```python
from build123d import *

# Parameters (mm, degrees)
F1_DEPTH = 50
F2_R     = 1.5
F3_DEPTH = 7
F4_R     = 1.5
F5_DEPTH = 7


with BuildPart() as f1:
    # F0 (on Front) → F1 (new body)
    with BuildSketch(Plane.XZ):
        Polygon((-2.165064, 1.25), (0, 0), (0, 2.5), align=None)
        Polygon((2.165064, -1.25), (0, 0), (0, -2.5), align=None)
        Polygon((0, 2.5), (0, 0), (2.165064, 1.25), align=None)
        Polygon((2.165064, 1.25), (0, 0), (2.165064, -1.25), align=None)
        Polygon((0, -2.5), (0, 0), (-2.165064, -1.25), align=None)
        Polygon((-2.165064, -1.25), (0, 0), (-2.165064, 1.25), align=None)
    extrude(amount=F1_DEPTH)

    # F2 (on face) → F3 (join)
    with BuildSketch(Plane.XZ.offset(50)):
        Circle(F2_R)
    extrude(amount=F3_DEPTH)

    # F4 (on face) → F5 (cut)
    with BuildSketch(Plane(origin=(0, 0, 0), x_dir=(-1, 0, 0), z_dir=(0, 1, 0))):
        Circle(F4_R)
    extrude(amount=-F5_DEPTH, mode=Mode.SUBTRACT)


solid = f1.part
```
Build history of the part. All positions in model axes, mm. A direction names the side the tool comes from. Round coordinates to 2 decimals unless told otherwise and drop trailing zeros. Loops run counter-clockwise (first coordinate to the right, second up) from the corner with the lowest first, then second, coordinate; pieces in that order, holes last.
Item 1: Which spindle directions (+Z, -Z, +X, -X, +Y, -Y) get a long thin tool onto all of the face, cutting with end or side? Do faces 1 (the face through (1.5, -3.45, 0.07)), 2 (the face through (-1.5, -53.45, 0.07)), 3 (the face through (1.07, -24.65, -1.88)). Say none if no direction does.
Item 2: Two-plate mould, pull along X, no slides. Class faces 4 (the face through (-1.07, -24.65, 1.88)), 5 (the face through (0, -7, 0)), 6 (the face through (0, -50, -2)): released by +X, released by -X, zero draft, split by the parting line, or undercut.
Item 3: Pin check, flat tip, straight feed: P1, Ø1.8, axis at x = 0, z = 0, coming from the +Y side. Stop position of the tip, or through.
Item 4: Saw through at B-B (y = -6). List the corners of the cut face in (x, z).
Item 5: Saw through at C-C (y = -46.5). List the corners of the cut face in (x, z).
Item 6: Drill centre lines: line 1 along Z through (x, y) = (0, -4.5); line 2 along Y through (x, z) = (0.15, 1.05); line 3 along Y through (x, z) = (0, -2.3). Where is each one in solid material? Low to high.
Item 7: Saw through at D-D (x = -0.9). List the corners of the cut face in (y, z).
Item 8: Saw through at A-A (z = 0). List the corners of the cut face in (x, y).
Worked answers:
1. face 1: +Y
1. face 2: -Y
1. face 3: -Z, +X, +Y, -Y
2. face 4: released by -X
2. face 5: undercut
2. face 6: zero draft
3. P1: stops at y = -7
4. outline: (-2.17, -1.25) - (0, -2.5) - (2.17, -1.25) - (2.17, 1.25) - (0, 2.5) - (-2.17, 1.25) - close; hole circle Ø3 at (0, 0)
5. outline: (-2.17, -1.25) - (0, -2.5) - (2.17, -1.25) - (2.17, 1.25) - (0, 2.5) - (-2.17, 1.25) - close
6. line 1: z = -2.5 to -1.5, 1.5 to 2.5
6. line 2: y = -57 to -7
6. line 3: y = -50 to 0
7. outline: (-57, -1.2) - (-50, -1.2) - (-50, -1.98) - (0, -1.98) - (0, -1.2) - (-7, -1.2) - (-7, 1.2) - (0, 1.2) - (0, 1.98) - (-50, 1.98) - (-50, 1.2) - (-57, 1.2) - close
8. outline: (-2.17, -50) - (-1.5, -50) - (-1.5, -57) - (1.5, -57) - (1.5, -50) - (2.17, -50) - (2.17, 0) - (1.5, 0) - (1.5, -7) - (-1.5, -7) - (-1.5, 0) - (-2.17, 0) - close
